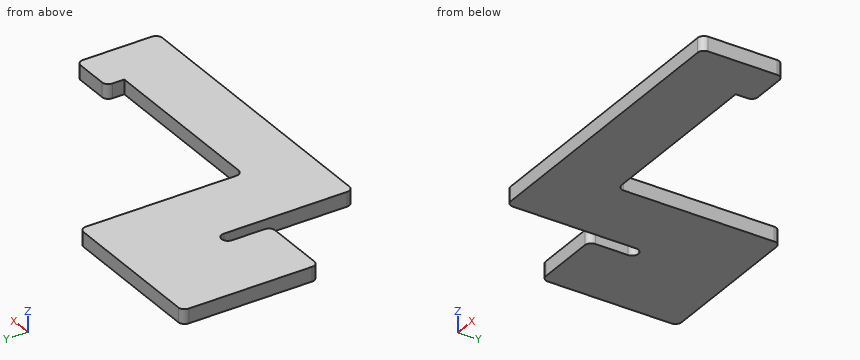
from build123d import *

# Parameters (mm, degrees)
F1_DEPTH = 2.032
F2_R     = 0.88899


# Not quite as in the source:
# - a fillet or chamfer is up to 0.001 mm smaller than in the source, because OpenCascade refuses the exact size


with BuildPart() as f1:
    # F0 (on Top) → F1 (new body)
    with BuildSketch(Plane.XY):
        Polygon((11.938, 12.7), (-10.16, 12.7), (-10.16, -6.35), (0, -6.35), (0, 0), (1.778, 0), (1.778, -19.05), (43.688, -19.05), (43.688, -7.62), (37.338, -7.62), (37.338, -10.16), (11.938, -10.16), align=None)
    extrude(amount=F1_DEPTH)

    # F2 (radius 0.889 in the source; OpenCascade refuses exactly that, so slightly less here)
    f2_edges = [f1.edges().sort_by_distance(p)[0] for p in [
        (-10.16, -6.35, 1.016),
        (0, -6.35, 1.016),
        (0, 0, 1.016),
        (1.778, 0, 1.016),
        (1.778, -19.05, 1.016),
        (-10.16, 12.7, 1.016),
        (37.338, -7.62, 1.016),
        (43.688, -19.05, 1.016),
        (11.938, 12.7, 1.016),
        (11.938, -10.16, 1.016),
        (43.688, -7.62, 1.016),
    ]]
    fillet(f2_edges, radius=F2_R)


solid = f1.part
Geometry check sheet. Reference: the model listing, model coordinates, mm. Round coordinates to 2 decimals unless told otherwise and drop trailing zeros. Order: outer loops, then holes, each group sorted by start corner. A loop starts at its lowest first (then second) coordinate and runs counter-clockwise, first axis right, second up. Notation, with made-up numbers: (11.25, 60.5) -> (64.25, 60.5) arc R28 cw to (64.25, 78.5) -> close; hole circle Ø5 at (42.5, 1.25). An arc over 180 degrees is marked (long way). Use one line per item in the form item = value.
1. Cross-section at D-D, the plane x = -3. Enter the section's corners in (y, z).
Working result:
outline = (-6.35, 0) -> (12.7, 0) -> (12.7, 2.03) -> (-6.35, 2.03) -> close
2. Cross-section at C-C, the plane y = -15.5. Enter the section's corners in (x, z), plus the area to 3 significant figures.
Working result:
outline = (1.78, 0) -> (43.69, 0) -> (43.69, 2.03) -> (1.78, 2.03) -> close
area = 85.2 mm^2
3. Cross-section at A-A, the plane y = -4.5. Enter the section's corners in (x, z).
Working result:
outline = (-10.16, 0) -> (0, 0) -> (0, 2.03) -> (-10.16, 2.03) -> close; (1.78, 0) -> (11.94, 0) -> (11.94, 2.03) -> (1.78, 2.03) -> close
4. Scan lines: line 1 along X through (y, z) = (-1, 0.6); line 2 along Y through (x, z) = (39.5, 1.6); line 3 along X through (y, z) = (-8.5, 1.45). Record each from-to range of solid material in increasing order. Write a range as from..to.
Working result:
line_1 = -10.16..0, 1.78..11.94
line_2 = -19.05..-7.62
line_3 = 1.78..11.94, 37.34..43.69
5. Go/stop test with flat-tipped pins: pin 1 (1 mm diameter, centred on x = 20, z = 1, fed in from +Y); pin 2 (1 mm diameter, centred on x = 41, z = 0.5, fed in from +Y). Record where each tip stops, or that it passes through.
Working result:
pin_1 = -10.16
pin_2 = -7.62
